Autodesk Inventor part; units mm, degrees
ref_plane "Work Plane2" through (0, 65, -37.4166) normal (0, 0, 1) x (1, 0, 0)
ref_plane "Work Plane3" through (0, 0, 0) normal (0, 1, 0) x (-1, 0, 0)
ref_plane "YZ Plane" through (0, 0, 0) normal (1, 0, 0) x (0, 1, 0)
sketch "Sketch11" plane through (0, 0, 0) normal (0, 0, 1) x (1, 0, 0)
  line L0 (-65, -65) -> (65, -65)
  line L1 (65, -65) -> (65, 65)
  line L2 (65, 65) -> (-65, 65)
  line L3 (-65, 65) -> (-65, -65)
  line L4 (-65, -65) -> (65, 65) construction
  line L5 (65, -65) -> (-65, 65) construction
  point P0 (0, 0)
  dimension "d36" = 130
  dimension "d37" = 130
extrude "Extrusion5" add sketch "Sketch11" against normal blind 150
sketch "Sketch12" plane through (0, 0, 0) normal (0, 0, 1) x (1, 0, 0)
  arc A0 (0, 75) -> (0, -75) centre (0, 0) ccw
  line L0 (0, 0) -> (0, 75) construction
  line L1 (0, 0) -> (75, 0) construction
  line L2 (0, 0) -> (0, -75) construction
  line L3 (0, 75) -> (0, -75)
  dimension "d40" = 75
  dimension "d41" = 90
  dimension "d42" = 180
revolve "Revolution5" cut sketch "Sketch12" angle 180 about axis through (0, 0, 0) along (0, -1, 0)
ref_plane "Work Plane2" through (0, 65, -37.4166) normal (0, 0, 1) x (1, 0, 0)
sketch "Sketch13" plane through (0, 65, -37.4166) normal (0, 0, 1) x (1, 0, 0)
  line L0 (-65, -130) -> (65, -130)
  line L1 (65, -130) -> (65, 0)
  line L2 (65, 0) -> (-65, 0)
  line L3 (-65, 0) -> (-65, -130)
  line L4 (-65, -130) -> (65, 0) construction
  line L5 (65, -130) -> (-65, 0) construction
  point P0 (0, -65)
  dimension "d45" = 130
  dimension "d46" = 130
extrude "Extrusion6" cut sketch "Sketch13" along normal blind 50
sketch "Sketch14" plane through (0, 65, -37.4166) normal (0, 0, 1) x (1, 0, 0)
  line L0 (-65, -130) -> (65, -130)
  line L1 (65, -130) -> (65, 0)
  line L2 (65, 0) -> (-65, 0)
  line L3 (-65, 0) -> (-65, -130)
  line L4 (-65, -130) -> (65, 0) construction
  line L5 (65, -130) -> (-65, 0) construction
  line L6 (-70, -135) -> (70, -135)
  line L7 (70, -135) -> (70, 5)
  line L8 (70, 5) -> (-70, 5)
  line L9 (-70, 5) -> (-70, -135)
  line L10 (-70, -135) -> (70, 5) construction
  line L11 (70, -135) -> (-70, 5) construction
  point P0 (0, -65)
  dimension "d49" = 130
  dimension "d50" = 130
  dimension "d51" = 140
  dimension "d52" = 140
extrude "Extrusion7" add sketch "Sketch14" against normal blind 75
sketch "Sketch17" plane through (0, 0, 0) normal (1, 0, 0) x (0, 1, 0)
  arc A0 (-80, 0) -> (80, 0) centre (0, 0) ccw
  line L0 (0, 0) -> (80, 0) construction
  line L1 (0, 0) -> (80, 0) construction
  line L2 (0, 0) -> (-80, 0) construction
  dimension "d57" = 80
  dimension "d58" = 0
  dimension "d59" = 180
sketch "Sketch18" plane through (-65, 65, -150) normal (0, 1, 0) x (1, 0, 0)
  line L0 (0, -37.5834) -> (130, -37.5834)
  line L1 (130, -37.5834) -> (130, 0)
  line L2 (130, 0) -> (0, 0)
  line L3 (0, 0) -> (0, -37.5834)
  point P0 (65, -150)
extrude "Extrusion9" cut sketch "Sketch18" against normal blind 140
ref_plane "Work Plane3" through (0, 0, 0) normal (0, 1, 0) x (-1, 0, 0)
sketch "Sketch22" plane through (0, 0, 0) normal (0, 1, 0) x (-1, 0, 0)
  arc A0 (-65, -37.4166) -> (65, -37.4166) centre (0, 0) ccw
  line L0 (0, -75) -> (0, 0)
  circle A1 centre (0, 0) radius 80
  circle A2 centre (0, 0) radius 150
  dimension "d74" = 160
  dimension "d75" = 300
extrude "Extrusion10" cut sketch "Sketch22" against normal blind 100 and the other way blind 100
sketch "Sketch24" plane through (0, 65, -37.4166) normal (0, 0, 1) x (1, 0, 0)
  circle A0 centre (-60.1041, -4.8959) radius 2
  point P0 (0, -65)
  dimension "d80" = 4
  dimension "d81" = 85
  dimension "d85" = 60.1041
sketch "Sketch25" plane through (0, 65, -37.4166) normal (0, 0, 1) x (1, 0, 0)
  circle A0 centre (60.1041, -4.8959) radius 2
  point P0 (0, -65)
  dimension "d82" = 4
  dimension "d83" = 85
  dimension "d84" = 60.1041
sketch "Sketch26" plane through (0, 65, -37.4166) normal (0, 0, 1) x (1, 0, 0)
  circle A0 centre (-60.1041, -125.1041) radius 2
  point P0 (0, -65)
  dimension "d86" = 4
  dimension "d87" = 85
  dimension "d88" = 60.1041
sketch "Sketch27" plane through (0, 65, -37.4166) normal (0, 0, 1) x (1, 0, 0)
  circle A0 centre (60.1041, -125.1041) radius 2
  point P0 (0, -65)
  dimension "d89" = 4
  dimension "d90" = 85
  dimension "d91" = 60.1041
hole "Hole1" at (-60.1041, 60.1041, -37.4166) direction (0, 0, -1) diameter 12.5 end through all
hole "Hole2" at (60.1041, 60.1041, -37.4166) direction (0, 0, -1) diameter 12.5 end through all
hole "Hole3" at (60.1041, -60.1041, -37.4166) direction (0, 0, -1) diameter 12.5 end through all
hole "Hole4" at (-60.1041, -60.1041, -37.4166) direction (0, 0, -1) diameter 12.5 end through all
equation "\"d37\" = d36"
equation "\"d46\" = d45"
properties part number "Custom Mirror Design"
Model file for the job. Use its own axes, mm. Give positions to 0.01 mm unless a question says otherwise; leave off trailing zeros. Loops run counter-clockwise (first coordinate to the right, second up) from the corner with the lowest first, then second, coordinate; pieces in that order, holes last. Notation, with made-up numbers: (-19.75, -16) - (26.25, -16) arc R21 ccw to (26.25, 20) - close; hole circle Ø3 at (44, 42). An arc over 180 degrees is marked (long way). One line per item, written item: value. Start each with the question number.
1. Slice it at B-B (z = -71.5). List the corners of the cut face in (x, y), plus the area to 3 significant figures.
2. Slice it at C-C (x = -28). List the corners of the cut face in (y, z), plus the area to 3 significant figures.
3. Slice it at A-A (y = -56). List the corners of the cut face in (x, z).
4. Slice it at D-D (y = 48.5). List the corners of the cut face in (x, z), plus the area to 3 significant figures.
5. Probe L1, parallel to X at y = -3, z = -41; L2, parallel to X at y = 11, z = -43; L3, parallel to Y at x = -4, z = -43.5. List the from-to ranges inside material, lowest first. Write a range as from..to.
6. Pin check, flat tips, straight feed: pin 1 (16 mm diameter, centred on x = 60.1, y = 60.1, fed in from -Z); pin 2 (3 mm diameter, centred on y = 50, z = -75.5, fed in from +X); pin 3 (12 mm diameter, centred on y = -6, z = -59, fed in from +X). Stop position of each tip, or through.
7. Pull direction Y, two halves, no side cores. Call faces 1 (the flat face through (1, 70, -54)), 2 (the flat face through (-1, -70, -54)), 3 (the cylindrical face through (-54.003, 61.459, -46.025)): pulls with the +Y half, pulls with the -Y half, needs draft (parallel to the pull), parting line crosses it, or undercut.
Solution:
1. outline: (-35.89, -70) - (35.89, -70) - (35.89, 70) - (-35.89, 70) - close; hole circle Ø45.29 at (0, 0)
1. area: 8,440 mm^2
2. outline: (-70, -74.94) - (70, -74.94) - (70, -37.42) - (58.66, -37.42) arc R69.58 cw to (-58.66, -37.42) - (-70, -37.42) - close
2. area: 2,590 mm^2
3. outline: (-70, -38.73) arc R80 ccw to (-64.82, -46.89) - (-64.82, -37.42) - (-70, -37.42) - close; (-55.39, -57.72) arc R80 ccw to (55.39, -57.72) - (55.39, -37.42) - (33, -37.42) arc R49.89 cw to (-33, -37.42) - (-55.39, -37.42) - close; (64.82, -46.89) arc R80 ccw to (70, -38.73) - (70, -37.42) - (64.82, -37.42) - close
4. outline: (-70, -38.73) arc R80 ccw to (70, -38.73) - (70, -37.42) - (43.28, -37.42) arc R57.21 cw to (-43.28, -37.42) - (-70, -37.42) - close
4. area: 3,100 mm^2
5. L1: x = -68.69..-62.73, 62.73..68.69
5. L2: x = -67.46..-60.46, 60.46..67.46
5. L3: y = -70..-60.97, 60.97..70
6. pin 1: stops at z = -60.71
6. pin 2: stops at x = 30.4
6. pin 3: stops at x = 59.92
7. face 1: pulls with the +Y half
7. face 2: pulls with the -Y half
7. face 3: undercut
